Part model, mm, in its own coordinate system. Face numbers are marked on the shaded views. A direction names the side the tool comes from. Give positions to 0.01 mm unless a question says otherwise; leave off trailing zeros. Order: outer loops, then holes, each group sorted by start corner. A loop starts at its lowest first (then second) coordinate and runs counter-clockwise, first axis right, second up. Notation, with made-up numbers: (49.5, 69.25) - (83.5, 69.25) arc R27 ccw to (83.5, 91.25) - close; hole circle Ø8 at (-33.5, -30.5). An arc over 180 degrees is marked (long way). One line per item, written item: value.
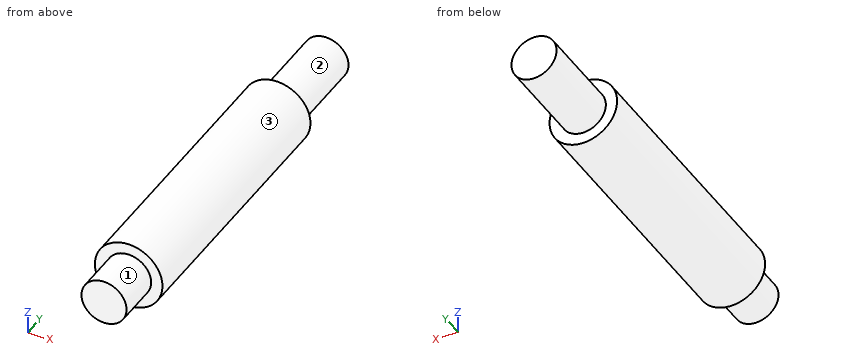
```python
from build123d import *

# Parameters (mm, degrees)
F0_R     = 9.525
F0_R_2   = 6.35
F1_DEPTH = 114.3
F2_R     = 9.525
F2_R_2   = 6.35
F3_DEPTH = 12.7
F4_R     = 9.525
F4_R_2   = 6.35
F5_DEPTH = 25.4


with BuildPart() as f1:
    # F0 (on Front) → F1 (new body)
    with BuildSketch(Plane.XZ):
        Circle(F0_R)
        Circle(F0_R_2, mode=Mode.SUBTRACT)
        Circle(F0_R_2)
    extrude(amount=F1_DEPTH)

    # F2 (on face) → F3 (cut)
    with BuildSketch(Plane.XZ.offset(114.3)):
        Circle(F2_R)
        Circle(F2_R_2, mode=Mode.SUBTRACT)
    extrude(amount=-F3_DEPTH, mode=Mode.SUBTRACT)

    # F4 (on face) → F5 (cut)
    with BuildSketch(Plane(origin=(0, 0, 0), x_dir=(-1, 0, 0), z_dir=(0, 1, 0))):
        Circle(F4_R)
        Circle(F4_R_2, mode=Mode.SUBTRACT)
    extrude(amount=-F5_DEPTH, mode=Mode.SUBTRACT)


solid = f1.part
```
1) Cut at B-B, the plane z = 0. Give the cut face in (x, y) (3 decimals).
Outcome:
outline: (-9.525, -101.6) - (-6.35, -101.6) - (-6.35, -114.3) - (6.35, -114.3) - (6.35, -101.6) - (9.525, -101.6) - (9.525, -25.4) - (6.35, -25.4) - (6.35, 0) - (-6.35, 0) - (-6.35, -25.4) - (-9.525, -25.4) - close
2) Cut at C-C, the plane y = -46. Give the cut face in (x, z) (3 decimals), then the cut area to 3 significant figures.
Outcome:
outline: circle Ø19.05 at (0, 0)
area: 285 mm^2
3) Cut at A-A, the plane x = 0. Give the cut face in (y, z) (3 decimals), then the cut area to 3 significant figures.
Outcome:
outline: (-114.3, -6.35) - (-101.6, -6.35) - (-101.6, -9.525) - (-25.4, -9.525) - (-25.4, -6.35) - (0, -6.35) - (0, 6.35) - (-25.4, 6.35) - (-25.4, 9.525) - (-101.6, 9.525) - (-101.6, 6.35) - (-114.3, 6.35) - close
area: 1,940 mm^2
4) Which spindle directions (+Z, -Z, +X, -X, +Y, -Y) get a long thin tool onto all of the face, cutting with end or side? Do the marked faces 1, 2 and 3. Say none if no direction does.
Outcome:
face 1: -Y
face 2: +Y
face 3: +Y, -Y
5) Drill centre lines: line 1 along Z through (x, y) = (-0.5, -13); line 2 along Y through (x, z) = (8.5, 0.75); line 3 along Z through (x, y) = (0, -83) (3 decimals). Where is each one in solid material? Low to high. Write a range as from..to.
Outcome:
line 1: z = -6.33..6.33
line 2: y = -101.6..-25.4
line 3: z = -9.525..9.525
6) Pin check, flat tips, straight feed: pin 1 (9.5 mm diameter, centred on x = -2, z = 3.5, fed in from +Y); pin 2 (5 mm diameter, centred on x = -5.5, z = -7, fed in from -Y); pin 3 (5 mm diameter, centred on x = 0, y = -20.5, fed in from +Z); pin 4 (5 mm diameter, centred on y = -47, z = -4.5, fed in from -X). Stop position of each tip, or through.
Outcome:
pin 1: stops at y = 0
pin 2: stops at y = -101.6
pin 3: stops at z = 6.35
pin 4: stops at x = -9.31
